Part model, mm, in its own coordinate system. A direction names the side the tool comes from. Round coordinates to 2 decimals unless told otherwise and drop trailing zeros. Order: outer loops, then holes, each group sorted by start corner. A loop starts at its lowest first (then second) coordinate and runs counter-clockwise, first axis right, second up. Notation, with made-up numbers: (39, -7.75) - (92, -7.75) arc R4 ccw to (92, -3.75) - close; hole circle Ø3 at (18, -20.75). An arc over 180 degrees is marked (long way). Answer as a JSON object with one key per item and string values.
```python
from build123d import *

# Parameters (mm, degrees)
F1_DEPTH = 65
F2_T     = -3
F4_DEPTH = 25


with BuildPart() as f1:
    # F0 (on Front) → F1 (new body)
    with BuildSketch(Plane.XZ):
        Polygon((13.628195, 74.95626), (-51.371805, 74.95626), (-79.687228, 14.233638), (-50.316361, -45.985563), (12.572752, -45.985563), (41.943619, 14.233638), align=None)
    extrude(amount=F1_DEPTH)

    # F2
    f2_openings = [f1.faces().sort_by_distance(p)[0] for p in [
        (-18.871805, -32.5, 74.95626),
    ]]
    offset(amount=F2_T, openings=f2_openings)

    # F3 (on face) → F4 (cut)
    with BuildSketch(Plane.XZ.offset(65)):
        with BuildLine():
            ThreePointArc((-46.871805, 74.95626), (-44.675105, 69.652959), (-39.371805, 67.45626))
            Line((-39.371805, 67.45626), (1.628195, 67.45626))
            ThreePointArc((1.628195, 67.45626), (6.931496, 69.652959), (9.128195, 74.95626))
            Line((9.128195, 74.95626), (-46.871805, 74.95626))
        make_face()
    extrude(amount=-F4_DEPTH, mode=Mode.SUBTRACT)


solid = f1.part
```
Item 1: Tool access for faces 5 (the flat face through (-19, -64, 67.456)), 6 (the flat face through (-62.6, -32.09, -13.96)), 7 (the flat face through (-65.21, -32.04, -15.45)): list every direction of +Z, -Z, +X, -X, +Y, -Y with a clear straight run to the whole face (end or side of a thin tool).
Taken from the geometry:
{"face 5": "+Z, -Y", "face 6": "none", "face 7": "-Z, -X, +Y, -Y"}
Item 2: Drop flat-ended pins along their axis: P1, Ø6, axis at y = -48.5, z = -13, coming from the +X side; P2, Ø4, axis at x = -59, y = -22, coming from the +Z side; P3, Ø3.5, axis at x = -17.5, y = -64, coming from the +Z side. Give the stop position or say it passes through.
Taken from the geometry:
{"P1": "x = 30.12", "P2": "z = 62.89", "P3": "z = 67.46"}
Item 3: Cut at B-B (y = -20). Write the cut outline in (x, z), plus the area to 3 significant figures.
Taken from the geometry:
{"outline": "(-79.69, 14.23) - (-50.32, -45.99) - (12.57, -45.99) - (41.94, 14.23) - (13.63, 74.96) - (10.32, 74.96) - (38.62, 14.26) - (10.7, -42.99) - (-48.44, -42.99) - (-76.36, 14.26) - (-48.06, 74.96) - (-51.37, 74.96) - close", "area": "977 mm2"}
Item 4: Cut at A-A (z = -7.5). Write the cut outline in (x, y).
Taken from the geometry:
{"outline": "(-69.09, -65) - (31.34, -65) - (31.34, 0) - (-69.09, 0) - close; hole (-65.75, -62) - (28.01, -62) - (28.01, -3) - (-65.75, -3) - close"}
Item 5: Probe L1, parallel to Y at x = -5.5, z = 53; L2, parallel to X at y = -32, z = 44; L3, parallel to X at y = -11, z = 6. List the from-to ranges inside material, lowest first. Write a range as from..to.
Taken from the geometry:
{"L1": "-65..-62, -3..0", "L2": "-65.81..-62.5, 24.75..28.06", "L3": "-75.67..-72.33, 34.59..37.93"}
Item 6: Cut at C-C (x = 21). Write the cut outline in (y, z), plus the area to 3 significant figures.
Taken from the geometry:
{"outline": "(-65, -28.71) - (0, -28.71) - (0, 59.15) - (-65, 59.15) - close; hole (-62, -21.86) - (-3, -21.86) - (-3, 52.05) - (-62, 52.05) - close", "area": "1,350 mm2"}
Item 7: Cut at D-D (x = -24). Write the cut outline in (y, z).
Taken from the geometry:
{"outline": "(-65, -45.99) - (0, -45.99) - (0, 74.96) - (-3, 74.96) - (-3, -42.99) - (-62, -42.99) - (-62, 67.46) - (-65, 67.46) - close"}
Item 8: Two-plate mould, pull along Y, no slides. Class faces 1 (the flat face through (-19, -32, -42.986)), 2 (the cylindrical face through (-45, -64, 70)), 3 (the flat face through (-20, 0, 15)), 4 (the flat face through (-62.015, -32.087, 45.034)): pulls with the +Y half, pulls with the -Y half, needs draft (parallel to the pull), parting line crosses it, or undercut.
Taken from the geometry:
{"face 1": "undercut", "face 2": "needs draft", "face 3": "pulls with the +Y half", "face 4": "undercut"}
